Source: CAD feature listing. Evaluate the final solid. Frame: model axes, mm. A direction names the side the tool comes from. Round coordinates to 2 decimals unless told otherwise and drop trailing zeros. Write each loop counter-clockwise with the first axis right and the second up, starting at its lowest first coordinate (ties: lowest second). Pieces come first, ordered by that corner, then holes. Notation, with made-up numbers: M -7.5,-26 L 36.5,-26 A26 cw 36.5,2 Z; hole C -15,34 d7. An arc over 180 degrees is marked long. Answer in a Markdown table with one row per item. Add a question column.
Item 1: Material intervals for probe 1 along X at (y, z) = (-1.65, -2); probe 2 along Y at (x, z) = (28, -15.5); probe 3 along Y at (x, z) = (37, -4), sorted ascending.
Item 2: Mould query, pull axis X, two halves, no side actions, for faces 1 (the face through (50.3, -4, -26)), 2 (the face through (37, -2, -53.48)). Classes: released by +X, released by -X, zero draft, split by the parting line, or undercut.
Item 3: Cut plane A-A on x = 2. Return loops of the section in (y, z), and give its area (3 significant figures).
Item 4: Set-up query: faces 3 (the face through (70, -1, -43)), 4 (the face through (10.3, -4, -26)), 5 (the face through (36, 0, -27)). Return all of +Z, -Z, +X, -X, +Y, -Y with unobstructed straight access to the full face (end or side cutting, diameter ignored); none if empty.
Item 5: Contact query for flat-ended pins moving along their axis: pin 1 (3 mm diameter, centred on y = -5, z = -25.5, fed in from -X); pin 2 (2.5 mm diameter, centred on x = 39, z = -23.5, fed in from -Y); pin 3 (1.3 mm diameter, centred on x = 2, z = -51.48, fed in from -Y). Output: stop coordinate, or through.
Item 6: Cut plane B-B on y = -4.1. Give the number of separate pieces and of enclosed holes in the cut face, and give its area (3 significant figures).
from build123d import *

# Parameters (mm, degrees)
EXTRUDE_2_DEPTH     = 6
SKETCH_1_6_W        = 4.5
SKETCH_1_6_H        = 3.99
CUT_EXTRUDE_1_DEPTH = 1
SKETCH_1_7_R        = 0.8
CUT_EXTRUDE_2_DEPTH = 6
SKETCH_1_8_R        = 0.8
CUT_EXTRUDE_3_DEPTH = 6
SKETCH_2_W          = 3
SKETCH_2_H          = 3.5
CUT_EXTRUDE_5_DEPTH = 60
FILLET_1_R          = 0.5


with BuildPart() as part:
    # Sketch 1 → Extrude 2 (new body)
    with BuildSketch(Plane(origin=(0, 0, 0), x_dir=(1, 0, 0), z_dir=(0, 1, 0))):
        Polygon((0, 0), (72.63, 0), (72.63, 40.8), (72.63, 44.79), (72.63, 53.48), (0, 53.48), align=None)
    extrude(amount=-EXTRUDE_2_DEPTH)

    # Sketch 1_6 → Cut-Extrude 1 (cut)
    with BuildSketch(Plane(origin=(0, 0, 0), x_dir=(1, 0, 0), z_dir=(0, 1, 0))):
        with Locations((70.38, 42.795)):
            Rectangle(SKETCH_1_6_W, SKETCH_1_6_H)
    extrude(amount=-CUT_EXTRUDE_1_DEPTH, mode=Mode.SUBTRACT)

    # Sketch 1_7 → Cut-Extrude 2 (cut)
    with BuildSketch(Plane(origin=(0, 0, 0), x_dir=(1, 0, 0), z_dir=(0, 1, 0))):
        with Locations(Location((2, 2, 0), (0, 0, 270))):
            Circle(SKETCH_1_7_R)
        with Locations(Location((70.879, 2, 0), (0, 0, 270))):
            Circle(SKETCH_1_7_R)
        with Locations(Location((2, 51.48, 0), (0, 0, 270))):
            Circle(SKETCH_1_7_R)
        with Locations(Location((70.879, 51.48, 0), (0, 0, 270))):
            Circle(SKETCH_1_7_R)
    extrude(amount=-CUT_EXTRUDE_2_DEPTH, mode=Mode.SUBTRACT)

    # Sketch 1_8 → Cut-Extrude 3 (cut)
    with BuildSketch(Plane(origin=(0, 0, 0), x_dir=(1, 0, 0), z_dir=(0, 1, 0))):
        with Locations(Location((2, 26.74, 0), (0, 0, 270))):
            Circle(SKETCH_1_8_R)
        with Locations(Location((70.879, 26.74, 0), (0, 0, 270))):
            Circle(SKETCH_1_8_R)
    extrude(amount=-CUT_EXTRUDE_3_DEPTH, mode=Mode.SUBTRACT)

    # Sketch 2 → Cut-Extrude 5 (cut)
    with BuildSketch(Plane.XY):
        with Locations((8.8, -4.25)):
            Rectangle(SKETCH_2_W, SKETCH_2_H)
        with Locations((13.8, -4.25)):
            Rectangle(SKETCH_2_W, SKETCH_2_H)
        with Locations((18.8, -4.25)):
            Rectangle(SKETCH_2_W, SKETCH_2_H)
        with Locations((23.8, -4.25)):
            Rectangle(SKETCH_2_W, SKETCH_2_H)
        with Locations((28.8, -4.25)):
            Rectangle(SKETCH_2_W, SKETCH_2_H)
        with Locations((33.8, -4.25)):
            Rectangle(SKETCH_2_W, SKETCH_2_H)
        with Locations((38.8, -4.25)):
            Rectangle(SKETCH_2_W, SKETCH_2_H)
        with Locations((43.8, -4.25)):
            Rectangle(SKETCH_2_W, SKETCH_2_H)
        with Locations((48.8, -4.25)):
            Rectangle(SKETCH_2_W, SKETCH_2_H)
        with Locations((53.8, -4.25)):
            Rectangle(SKETCH_2_W, SKETCH_2_H)
        with Locations((58.8, -4.25)):
            Rectangle(SKETCH_2_W, SKETCH_2_H)
        with Locations((63.8, -4.25)):
            Rectangle(SKETCH_2_W, SKETCH_2_H)
    extrude(amount=-CUT_EXTRUDE_5_DEPTH, mode=Mode.SUBTRACT)

    # Fillet 1
    fillet_1_edges = [part.edges().sort_by_distance(p)[0] for p in [
        (62.3, -6, -26.74),
        (57.3, -6, -26.74),
        (60.3, -6, -26.74),
        (52.3, -6, -26.74),
        (55.3, -6, -26.74),
        (47.3, -6, -26.74),
        (50.3, -6, -26.74),
        (42.3, -6, -26.74),
        (45.3, -6, -26.74),
        (37.3, -6, -26.74),
        (40.3, -6, -26.74),
        (32.3, -6, -26.74),
        (35.3, -6, -26.74),
        (27.3, -6, -26.74),
        (30.3, -6, -26.74),
        (22.3, -6, -26.74),
        (25.3, -6, -26.74),
        (17.3, -6, -26.74),
        (20.3, -6, -26.74),
        (12.3, -6, -26.74),
        (15.3, -6, -26.74),
        (10.3, -6, -26.74),
    ]]
    fillet(fillet_1_edges, radius=FILLET_1_R)


solid = part.part
Results below:
| question | item | result |
|---|---|---|
| 1 | probe 1 | 0 to 1.2, 2.8 to 70.08, 71.68 to 72.63 |
| 1 | probe 2 | -2.5 to 0 |
| 1 | probe 3 | -5.96 to 0 |
| 2 | face 1 | undercut |
| 2 | face 2 | zero draft |
| 3 | outline | M -6,-53.48 L 0,-53.48 L 0,-52.28 L -6,-52.28 Z; M -6,-50.68 L 0,-50.68 L 0,-27.54 L -6,-27.54 Z; M -6,-25.94 L 0,-25.94 L 0,-2.8 L -6,-2.8 Z; M -6,-1.2 L 0,-1.2 L 0,0 L -6,0 Z |
| 3 | area | 292 mm2 |
| 4 | face 3 | +X, +Y |
| 4 | face 4 | +Z, -Z, -Y |
| 4 | face 5 | +Z, -Z, +X, -X, +Y |
| 5 | pin 1 | x = 0 |
| 5 | pin 2 | y = -2.5 |
| 5 | pin 3 | through |
| 6 | separate pieces | 13 |
| 6 | enclosed holes | 6 |
| 6 | area | 1,950 mm2 |
